```python
from build123d import *

# Parameters (mm, degrees)
SKETCH1_W                  = 139.7
SKETCH1_H                  = 139.7
EXTRUDE1_DEPTH             = 9.525
F_1_2_0_5_DIAMETER_HOLE1_D = 12.7
CIRPATTERN1_COUNT          = 4


with BuildPart() as part:
    # Sketch1 → Extrude1 (new body)
    with BuildSketch(Plane.XY):
        Rectangle(SKETCH1_W, SKETCH1_H)
    extrude(amount=EXTRUDE1_DEPTH)

    # 1_2 _0.5_ Diameter Hole1 (through all)
    with Locations(Plane(origin=(-33.226947648, 33.226947648, 9.525), x_dir=(1, 0, 0), z_dir=(0, 0, 1))):
        with Locations((0, 0)):
            f_1_2_0_5_diameter_hole1 = Hole(F_1_2_0_5_DIAMETER_HOLE1_D / 2)

    # Sketch4 → D _0.246_ Diameter Hole1 (revolve, cut)
    with BuildSketch(Plane(origin=(-56.0324, 11.43, 9.525), x_dir=(0, -1, 0), z_dir=(1, 0, 0))):
        Polygon((0, 0), (0, 35.659208746), (3.1242, 33.782), (3.1242, 0), align=None)
    d_0_246_diameter_hole1 = revolve(axis=Axis((-56.0324, 11.43, 15.875), (0, 0, -1)), mode=Mode.SUBTRACT)

    # Sketch5 → 1_4 _0.25_ Diameter Hole1 (revolve, cut)
    with BuildSketch(Plane(origin=(-56.0324, -11.43, 9.525), x_dir=(0, -1, 0), z_dir=(1, 0, 0))):
        Polygon((0, 0), (0, 35.689732465), (3.175, 33.782), (3.175, 0), align=None)
    f_1_4_0_25_diameter_hole1 = revolve(axis=Axis((-56.0324, -11.43, 15.875), (0, 0, -1)), mode=Mode.SUBTRACT)

    # CirPattern1: 1_2 _0.5_ Diameter Hole1, D _0.246_ Diameter Hole1, 1_4 _0.25_ Diameter Hole1 ×4 about axis
    cirpattern1_axis = Axis((0, 0, 0), (0, 0, 1))
    for i in range(1, CIRPATTERN1_COUNT):
        add(f_1_2_0_5_diameter_hole1.rotate(cirpattern1_axis, i * 360 / CIRPATTERN1_COUNT), mode=Mode.SUBTRACT)
        add(d_0_246_diameter_hole1.rotate(cirpattern1_axis, i * 360 / CIRPATTERN1_COUNT), mode=Mode.SUBTRACT)
        add(f_1_4_0_25_diameter_hole1.rotate(cirpattern1_axis, i * 360 / CIRPATTERN1_COUNT), mode=Mode.SUBTRACT)


solid = part.part
```
The listing builds one solid part. Answer for the finished solid, in the listing's coordinates (mm). Coordinates: 2 decimals unless noted, no trailing zeros. Write each loop counter-clockwise with the first axis right and the second up, starting at its lowest first coordinate (ties: lowest second). Pieces come first, ordered by that corner, then holes. Notation, with made-up numbers: (52.25, 58.25) -> (108.25, 58.25) arc R20 cw to (108.25, 95.25) -> close; hole circle Ø9 at (37, 30). An arc over 180 degrees is marked (long way). Write each question's results on one line, items separated by ' | '. Start each with the question number.
1) Straight lines are drawn through the part: probe 1 along Y at (x, z) = (11.43, 7); probe 2 along Y at (x, z) = (35, 6.5); probe 3 along X at (y, z) = (11.43, 4.25). For each, find the intervals that lie inside material, in ascending order.
2) A flat-ended cylindrical pin translates along its axis: pin 1 Ø3.5 at (x, y) = (-11.43, -56.03) entering from +Z. Find the tip coordinate at first contact, or state that the pin passes through.
3) A cutting plane is placed at A-A (y = -11.43). Determine the outline of the cut face in (x, z) (3 decimals), then the cut area to 3 significant figures.
4) For a pull along Y with two mould halves and no side action, classify faces 1 (the cylindrical face through (-31.85, 27.03, 4.7)), 2 (the flat face through (-1, 69.85, 5)), 3 (the flat face through (-1, 1, 0)) as +Y half, -Y half, draft (parallel to the pull), parting line (faces both ways), or undercut.
5) A cutting plane is placed at C-C (z = 3.5). Count the separate pieces of the cut face and the enclosed holes in it, then the cut area to 3 significant figures.
Values follow:
1) probe 1: -69.85 to -59.21, -52.86 to 52.91, 59.16 to 69.85 | probe 2: -69.85 to -39.32, -27.13 to 27.13, 39.32 to 69.85 | probe 3: -69.85 to -59.16, -52.91 to 52.86, 59.21 to 69.85
2) pin 1: through
3) outline: (-69.85, 0) -> (-59.207, 0) -> (-59.207, 9.525) -> (-69.85, 9.525) -> close; (-52.857, 0) -> (52.908, 0) -> (52.908, 9.525) -> (-52.857, 9.525) -> close; (59.157, 0) -> (69.85, 0) -> (69.85, 9.525) -> (59.157, 9.525) -> close | area: 1,210 mm²
4) face 1: undercut | face 2: +Y half | face 3: draft
5) separate pieces: 1 | enclosed holes: 12 | area: 18,800 mm²
